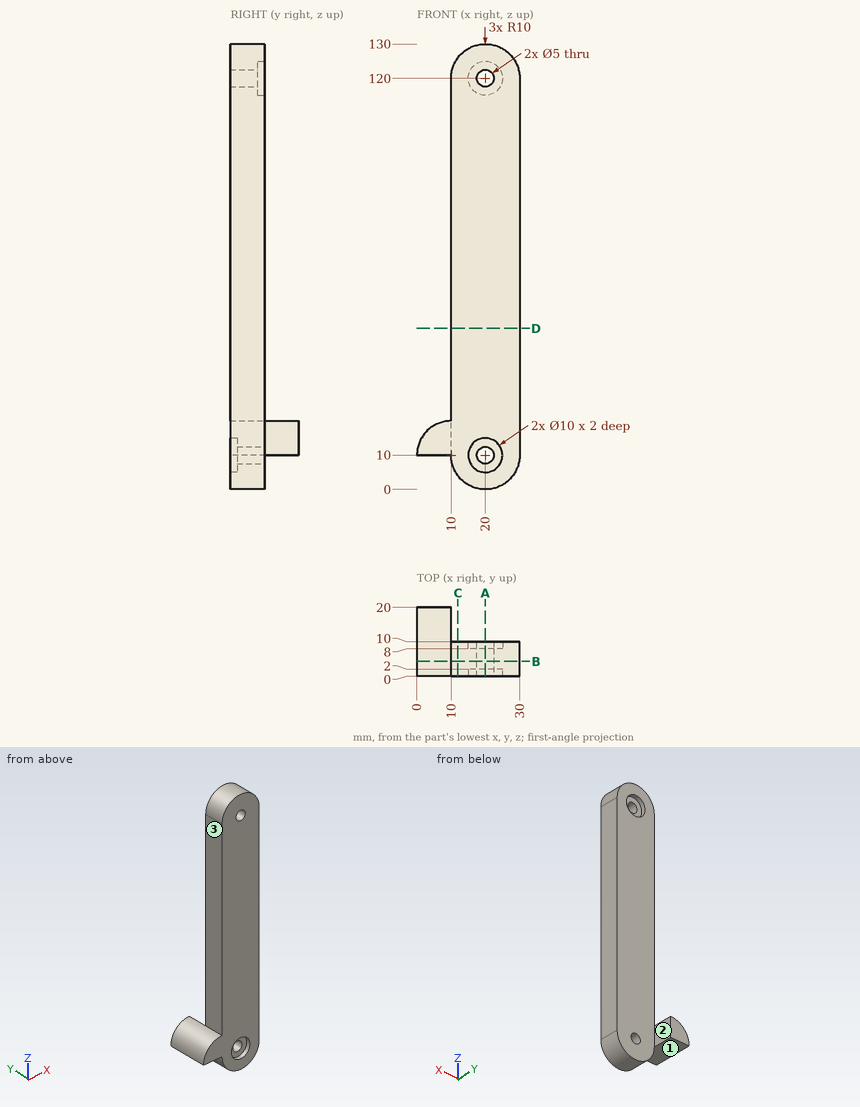
Check sheet for the drawn part. Datum: minimum x, y, z corner. Units: mm. A direction names the side the tool comes from. Round coordinates to 2 decimals unless told otherwise and drop trailing zeros. Order: outer loops, then holes, each group sorted by start corner. A loop starts at its lowest first (then second) coordinate and runs counter-clockwise, first axis right, second up.
1) Scan lines: line 1 (Z direction, x = 20, y = 0.75); line 2 (X direction, y = 3.25, z = 120); line 3 (Z direction, x = 22, y = 6). Record each from-to range of solid material in increasing order.
2) Section check B-B (y = 4.25). Record the boundary of the cut face in (x, z), and give its area (3 significant figures).
3) Go/stop test with flat-tipped pins: pin 1 Ø3 at (x, z) = (19.5, 9) entering from -Y; pin 2 Ø6 at (x, z) = (19.5, 62.5) entering from +Y; pin 3 Ø5 at (x, y) = (6, 5) entering from -Z. Record where each tip stops, or that it passes through.
4) Tool access check on the marked faces 1, 2 and 3. Record the directions out of +Z, -Z, +X, -X, +Y, -Y that give a thin tool (end or side, any length) a straight path to the whole face; none if there is none.
5) Section check A-A (x = 20). Record the boundary of the cut face in (y, z), and give its area (3 significant figures).
6) Section check C-C (x = 12). Record the boundary of the cut face in (y, z).
7) Section check D-D (z = 47). Record the boundary of the cut face in (x, y), and give its area (3 significant figures).
Result:
1. line 1: z = 0 to 5, 15 to 117.5, 122.5 to 130
1. line 2: x = 10 to 17.5, 22.5 to 30
1. line 3: z = 0.2 to 8.5, 11.5 to 118.5, 121.5 to 129.8
2. outline: (0, 10) - (10, 10) arc R10 ccw to (30, 10) - (30, 120) arc R10 ccw to (10, 120) - (10, 20) arc R10 ccw to start; hole circle Ø5 at (20, 10); hole circle Ø5 at (20, 120)
2. area: 2,550 mm2
3. pin 1: stops at y = 2
3. pin 2: stops at y = 10
3. pin 3: stops at z = 10
4. face 1: -Z, -X, +Y, -Y
4. face 2: +Z, -Z, +X, +Y
4. face 3: +Z, -X, +Y, -Y
5. outline: (0, 0) - (10, 0) - (10, 7.5) - (2, 7.5) - (2, 5) - (0, 5) - close; (0, 15) - (2, 15) - (2, 12.5) - (10, 12.5) - (10, 115) - (8, 115) - (8, 117.5) - (0, 117.5) - close; (0, 122.5) - (8, 122.5) - (8, 125) - (10, 125) - (10, 130) - (0, 130) - close
5. area: 1,180 mm2
6. outline: (0, 4) - (10, 4) - (10, 126) - (0, 126) - close
7. outline: (10, 0) - (30, 0) - (30, 10) - (10, 10) - close
7. area: 200 mm2
